Verification items for the finished model (mm, model axes). Face numbers are marked on the shaded views. A direction names the side the tool comes from. Coordinates: 2 decimals unless noted, no trailing zeros. Order: outer loops, then holes, each group sorted by start corner. A loop starts at its lowest first (then second) coordinate and runs counter-clockwise, first axis right, second up. Notation, with made-up numbers: (-3.5, 10) -> (47.5, 10) arc R27 cw to (47.5, 30) -> close; hole circle Ø5 at (19, -2.75). An arc over 180 degrees is marked (long way). Write each question's results on one line, items separated by ' | '. Start each with the question number.
(1) Thickness scan on probe 1 along Y at (x, z) = (7, -165); probe 2 along Z at (x, y) = (6, 179); probe 3 along X at (y, z) = (166, -31.5). Record the ranges inside material, lowest first. Write a range as [from, to].
(2) Cross-section at A-A on z = -45. Enter the section's corners in (x, y), and give its area (3 significant figures).
(3) Set-up check for the marked faces 1 and 2: record each of +Z, -Z, +X, -X, +Y, -Y from which the full face is reachable in a straight line by a thin tool's end or side.
(4) Cross-section at D-D on z = -153. Enter the section's corners in (x, y).
(5) Cross-section at B-B on x = 3. Enter the section's corners in (y, z).
(6) Go/stop test with flat-tipped pins: pin 1 (6 mm diameter, centred on x = -9.5, z = -36.5, fed in from +Y); pin 2 (11.5 mm diameter, centred on y = 180.81, z = -165, fed in from +X); pin 3 (6 mm diameter, centred on y = 185, z = -46.5, fed in from -X). Record where each tip stops, or that it passes through.
(7) Cross-section at C-C on y = 182. Enter the section's corners in (x, z), and give its area (3 significant figures).
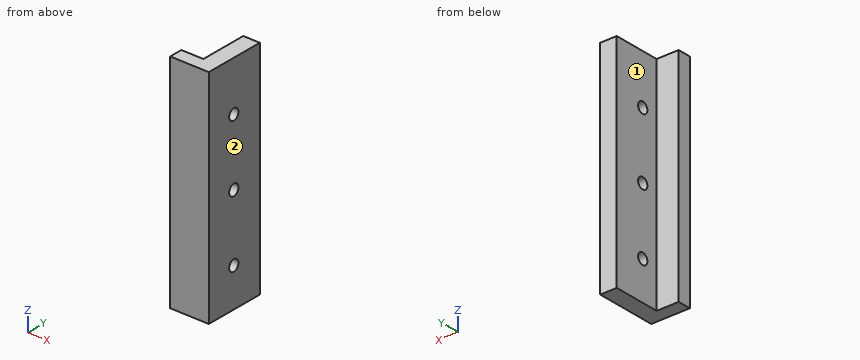
```python
from build123d import *

# Parameters (mm, degrees)
EXTRUDE_1_DEPTH                 = 200
CUT_EXTRUDE_1_REACH             = 293.247
SKETCH_2_R                      = 5
CUT_EXTRUDE_1_DIRECTION_2_DEPTH = 292.246667899


with BuildPart() as part:
    # 草圖1 → 填料-伸長1 (new body)
    with BuildSketch(Plane.XY):
        Polygon((-5.019605957, 208.805223982), (-5.019605957, 165.805223982), (-25.019605957, 165.805223982), (-25.019605957, 153.805223982), (9.980394043, 153.805223982), (9.980394043, 208.805223982), align=None)
    extrude(amount=-EXTRUDE_1_DEPTH)

    # 草圖2 → 除料-伸長1 (cut, up to next)
    with BuildSketch(Plane(origin=(9.980394043, 0, 0), x_dir=(0, 0, -1), z_dir=(1, 0, 0)), mode=Mode.PRIVATE) as cut_extrude_1_sk1:
        with Locations(Location((45, 180.805223982, 0), (0, 0, 270))):
            Circle(SKETCH_2_R)
    cut_extrude_1_tool1 = extrude(cut_extrude_1_sk1.sketch, amount=-CUT_EXTRUDE_1_REACH, mode=Mode.PRIVATE) & part.part
    # 草圖2 → 除料-伸長1 (cut, up to next)
    with BuildSketch(Plane(origin=(9.980394043, 0, 0), x_dir=(0, 0, -1), z_dir=(1, 0, 0)), mode=Mode.PRIVATE) as cut_extrude_1_sk2:
        with Locations(Location((105, 180.805223982, 0), (0, 0, 270))):
            Circle(SKETCH_2_R)
    cut_extrude_1_tool2 = extrude(cut_extrude_1_sk2.sketch, amount=-CUT_EXTRUDE_1_REACH, mode=Mode.PRIVATE) & part.part
    # 草圖2 → 除料-伸長1 (cut, up to next)
    with BuildSketch(Plane(origin=(9.980394043, 0, 0), x_dir=(0, 0, -1), z_dir=(1, 0, 0)), mode=Mode.PRIVATE) as cut_extrude_1_sk3:
        with Locations(Location((165, 180.805223982, 0), (0, 0, 270))):
            Circle(SKETCH_2_R)
    cut_extrude_1_tool3 = extrude(cut_extrude_1_sk3.sketch, amount=-CUT_EXTRUDE_1_REACH, mode=Mode.PRIVATE) & part.part
    add(cut_extrude_1_tool1.solids().sort_by_distance((9.980394, 180.805224, -45))[0], mode=Mode.SUBTRACT)
    add(cut_extrude_1_tool2.solids().sort_by_distance((9.980394, 180.805224, -105))[0], mode=Mode.SUBTRACT)
    add(cut_extrude_1_tool3.solids().sort_by_distance((9.980394, 180.805224, -165))[0], mode=Mode.SUBTRACT)

    # 草圖2 → 除料-伸長1 direction 2 (cut)
    with BuildSketch(Plane(origin=(9.980394043, 0, 0), x_dir=(0, 0, -1), z_dir=(1, 0, 0))):
        with Locations(Location((45, 180.805223982, 0), (0, 0, 270))):
            Circle(SKETCH_2_R)
        with Locations(Location((105, 180.805223982, 0), (0, 0, 270))):
            Circle(SKETCH_2_R)
        with Locations(Location((165, 180.805223982, 0), (0, 0, 270))):
            Circle(SKETCH_2_R)
    extrude(amount=CUT_EXTRUDE_1_DIRECTION_2_DEPTH, mode=Mode.SUBTRACT)


solid = part.part
```
Results are:
1) probe 1: y = [153.81, 175.81], [185.81, 208.81] | probe 2: z = [-200, -169.66], [-160.34, -109.66], [-100.34, -49.66], [-40.34, 0] | probe 3: x = [-5.02, 9.98]
2) outline: (-25.02, 153.81) -> (9.98, 153.81) -> (9.98, 175.81) -> (-5.02, 175.81) -> (-5.02, 165.81) -> (-25.02, 165.81) -> close; (-5.02, 185.81) -> (9.98, 185.81) -> (9.98, 208.81) -> (-5.02, 208.81) -> close | area: 915 mm2
3) face 1: +Z, -Z, -X, +Y | face 2: +Z, -Z, +X, +Y, -Y
4) outline: (-25.02, 153.81) -> (9.98, 153.81) -> (9.98, 208.81) -> (-5.02, 208.81) -> (-5.02, 165.81) -> (-25.02, 165.81) -> close
5) outline: (153.81, -200) -> (208.81, -200) -> (208.81, 0) -> (153.81, 0) -> close; hole circle Ø10 at (180.81, -165); hole circle Ø10 at (180.81, -105); hole circle Ø10 at (180.81, -45)
6) pin 1: stops at y = 165.81 | pin 2: stops at x = 9.98 | pin 3: stops at x = -5.02
7) outline: (-5.02, -200) -> (9.98, -200) -> (9.98, -169.86) -> (-5.02, -169.86) -> close; (-5.02, -160.14) -> (9.98, -160.14) -> (9.98, -109.86) -> (-5.02, -109.86) -> close; (-5.02, -100.14) -> (9.98, -100.14) -> (9.98, -49.86) -> (-5.02, -49.86) -> close; (-5.02, -40.14) -> (9.98, -40.14) -> (9.98, 0) -> (-5.02, 0) -> close | area: 2,560 mm2
